Geometry check sheet. Reference: the model listing, model coordinates, mm. A direction names the side the tool comes from. Round coordinates to 2 decimals unless told otherwise and drop trailing zeros. Loops run counter-clockwise (first coordinate to the right, second up) from the corner with the lowest first, then second, coordinate; pieces in that order, holes last. Notation, with made-up numbers: (26.5, -30) - (45.5, -30) arc R24 ccw to (45.5, 2) - close; hole circle Ø11 at (60, -6). An arc over 180 degrees is marked (long way). Answer in a Markdown table with one row per item. Add a question column.
```python
from build123d import *

# Parameters (mm, degrees)
SKETCH1_R                = 22
SKETCH1_R_2              = 16
BOSS_EXTRUDE1_DEPTH      = 20
BOSS_EXTRUDE2_REACH      = 55.774
BOSS_EXTRUDE2_END_RADIUS = 22
SKETCH5_W                = 20
SKETCH5_H                = 40
SKETCH6_R                = 5.25
BOSS_EXTRUDE3_DEPTH      = 10


with BuildPart() as part:
    # Sketch1 → Boss-Extrude1 (new, symmetric)
    with BuildSketch(Plane.XY):
        with Locations((0, 41.80685414)):
            Circle(SKETCH1_R)
        with Locations((0, 41.80685414)):
            Circle(SKETCH1_R_2, mode=Mode.SUBTRACT)
    extrude(amount=BOSS_EXTRUDE1_DEPTH, both=True)

    # Boss-Extrude2: up to this cylinder (the profile starts outside it)
    boss_extrude2_end = Plane(origin=(0, 41.80685414, 0), z_dir=(0, 0, -1)) * Cylinder(BOSS_EXTRUDE2_END_RADIUS, 156.548, mode=Mode.PRIVATE)
    # Sketch5 → Boss-Extrude2 (add, up to the surface)
    with BuildSketch(Plane(origin=(0, 19, 0), x_dir=(1, 0, 0), z_dir=(0, 1, 0)), mode=Mode.PRIVATE) as boss_extrude2_sk1:
        Rectangle(SKETCH5_W, SKETCH5_H)
    boss_extrude2_tool1 = extrude(boss_extrude2_sk1.sketch, amount=BOSS_EXTRUDE2_REACH, mode=Mode.PRIVATE) - boss_extrude2_end
    add(boss_extrude2_tool1.solids().sort_by_distance((0, 19, 0))[0])

    # Sketch6 → Boss-Extrude3 (add, symmetric)
    with BuildSketch(Plane(origin=(0, 0, 0), x_dir=(0, 0, -1), z_dir=(1, 0, 0))):
        with BuildLine():
            Line((-20, 19), (-15, 5.842729547))
            ThreePointArc((-15, 5.842729547), (0, -4.503591016), (15, 5.842729547))
            Line((15, 5.842729547), (20, 19))
            Line((20, 19), (-20, 19))
        make_face()
        with Locations((0, 6.293)):
            Circle(SKETCH6_R, mode=Mode.SUBTRACT)
    extrude(amount=BOSS_EXTRUDE3_DEPTH, both=True)


solid = part.part
```
Q1. Cross-section at C-C, the plane y = 33.5. Enter the section's corners in (x, z).
Q2. Release check for a two-part mould opening along Y. For faces 1 (the flat face through (0.14, 12.329, -17.465)), 2 (the flat face through (-10, 12, 0)), 3 (the cylindrical face through (-0.1, 7.9, -5)) record: +Y half, -Y half, draft (parallel to the pull), parting line (faces both ways), or undercut.
Q3. Scan lines: line 1 (Y direction, x = -1, z = 0); line 2 (Y direction, x = -2.25, z = 0); line 3 (Y direction, x = 0, z = 8.5). Record each from-to range of solid material in increasing order. Write a range as from..to.
Q4. Cross-section at D-D, the plane x = 11. Enter the section's corners in (y, z).
Q5. Depth check by flat-ended pin: P1, Ø3, axis at y = 50.5, z = -3.5, coming from the +X side; P2, Ø5, axis at x = 11, z = -6, coming from the +Y side; P3, Ø3, axis at x = -12, z = -1, coming from the -Y side; P4, Ø3, axis at x = -15, y = 24.5, coming from the -Z side. Enter the tip coordinate at first touch or a pass-through.
Q6. Cross-section at B-B, the plane z = 0. Enter the section's corners in (x, y).
Q7. Set-up check for faces 4 (the flat face through (0, 25, -20)), 5 (the flat face through (10, 12, 0)): record each of +Z, -Z, +X, -X, +Y, -Y from which the full face is reachable in a straight line by a thin tool's end or side.
Q8. Cross-section at A-A, the plane x = 0. Enter the section's corners in (y, z), plus the area to 3 significant figures.
Check sheet entries:
| question | item | result |
|---|---|---|
| 1 | outline | (-20.37, -20) - (-13.67, -20) - (-13.67, 20) - (-20.37, 20) - close; (13.67, -20) - (20.37, -20) - (20.37, 20) - (13.67, 20) - close |
| 2 | face 1 | -Y half |
| 2 | face 2 | draft |
| 2 | face 3 | undercut |
| 3 | line 1 | -4.5..1.04, 11.54..25.84, 57.78..63.78 |
| 3 | line 2 | -4.5..1.04, 11.54..25.97, 57.65..63.69 |
| 3 | line 3 | -2.07..25.81, 57.81..63.81 |
| 4 | outline | (22.75, -20) - (30.19, -20) - (30.19, 20) - (22.75, 20) - close; (53.43, -20) - (60.86, -20) - (60.86, 20) - (53.43, 20) - close |
| 5 | P1 | x = 20.79 |
| 5 | P2 | y = 62.1 |
| 5 | P3 | y = 22.47 |
| 5 | P4 | z = -20 |
| 6 | outline | (-10, -4.5) - (10, -4.5) - (10, 1.04) - (-10, 1.04) - close; (-10, 11.54) - (10, 11.54) - (10, 22.21) arc R22 ccw (long way) to (-10, 22.21) - close; hole circle Ø32 at (0, 41.81) |
| 7 | face 4 | -Z, +X, -X, +Y, -Y |
| 7 | face 5 | +Z, -Z, +X, -Y |
| 8 | outline | (5.84, -15) - (19, -20) - (25.81, -20) - (25.81, 20) - (19, 20) - (5.84, 15) arc R16.05 ccw to start; (57.81, -20) - (63.81, -20) - (63.81, 20) - (57.81, 20) - close; hole circle Ø10.5 at (6.29, 0) |
| 8 | area | 1,110 mm² |
